Could you check a few things on this model? Use its own coordinates, in mm. Face numbers are marked on the shaded views. A direction names the side the tool comes from. Coordinates: 2 decimals unless noted, no trailing zeros. Loops run counter-clockwise (first coordinate to the right, second up) from the corner with the lowest first, then second, coordinate; pieces in that order, holes last.
1) Will these pins go through, and if not, where does the flat tip stop? P1, Ø6, axis at x = 47, z = 15, coming from the -Y side; P2, Ø14.5, axis at y = -20.5, z = 7, coming from the -X side; P3, Ø6, axis at x = 19.5, y = -26.5, coming from the +Z side; P4, Ø4, axis at x = 47.5, z = 4.5, coming from the -Y side.
2) Thinking about a two-plate mould opening in X: for the marked faces 4, 5 and 6, which applies, released by +X, released by -X, zero draft, split by the parting line, or undercut?
3) Imagine slicing it at B-B on x = 20.5. Please give me the cut outline in (y, z), plus the area to 3 significant figures.
4) For the marked faces 1, 2 and 3, which set-ups out of +Z, -Z, +X, -X, +Y, -Y let a thin tool reach every point of the face, with its end or its side?
5) If I drill on line 1 along Y through (x, z) = (10.5, 13.5); line 2 along X through (y, z) = (-9, 4.5); line 3 along X through (y, z) = (-27.5, -0.5), over which ranges is the centre line in solid material (lowest first)?
6) Imagine slicing it at D-D on y = -20. Please give me the cut outline in (x, z).
7) Imagine slicing it at C-C on z = -0.5. Please give me the cut outline in (x, y).
```python
from build123d import *

# Parameters (mm, degrees)
F0_W     = 52
F0_H     = 32
F1_DEPTH = 40
F2_R     = 15.99999
F3_R     = 8
F4_DEPTH = 40.001
F5_W     = 26.99999
F5_H     = 18
F5_W_2   = 25.00001
F6_DEPTH = 32.001
F7_R     = 9
F8_DEPTH = 32


# Not quite as in the source:
# - a fillet or chamfer is up to 0.001 mm smaller than in the source, because OpenCascade refuses the exact size


with BuildPart() as f1:
    # F0 (on Front) → F1 (new body)
    with BuildSketch(Plane.XZ):
        with Locations((6.3565019518, 4.5450745088)):
            Rectangle(F0_W, F0_H)
    extrude(amount=F1_DEPTH)

    # F2 (radius 16 in the source; OpenCascade refuses exactly that, so slightly less here)
    f2_edges = [f1.edges().sort_by_distance(p)[0] for p in [
        (-19.643498, -20, 20.545075),
        (-19.643498, -20, -11.454925),
    ]]
    fillet(f2_edges, radius=F2_R)

    # F3 (on face) → F4 (cut, through all)
    with BuildSketch(Plane.XZ.offset(40)):
        with Locations((-3.6434980482, 4.5450745088)):
            Circle(F3_R)
    extrude(amount=-F4_DEPTH, mode=Mode.SUBTRACT)

    # F5 (on face) → F6 (cut, through all)
    with BuildSketch(Plane.XY.offset(20.5450745088)):
        with Locations((-17.1435030482, -20)):
            Rectangle(F5_W, F5_H)
        with Locations((8.8564969518, -20)):
            Rectangle(F5_W_2, F5_H)
    extrude(amount=-F6_DEPTH, mode=Mode.SUBTRACT)

    # F7 (on face) → F8 (join)
    with BuildSketch(Plane.YZ.offset(32.3565019518)):
        with Locations((-20, 4.5450745088)):
            Circle(F7_R)
    extrude(amount=F8_DEPTH)


solid = f1.part
```
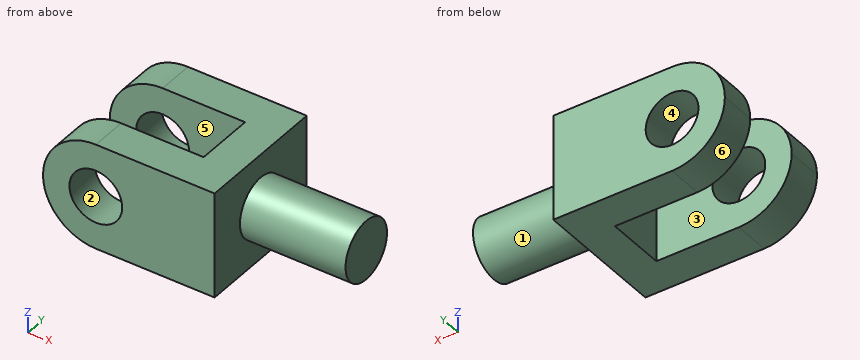
Filled in:
1. P1: stops at y = -25.04
1. P2: stops at x = 21.36
1. P3: stops at z = 20.55
1. P4: stops at y = -29
2. face 4: undercut
2. face 5: zero draft
2. face 6: released by -X
3. outline: (-40, -11.45) - (-29, -11.45) - (-29, 20.55) - (-40, 20.55) - close; (-11, -11.45) - (0, -11.45) - (0, 20.55) - (-11, 20.55) - close
3. area: 704 mm2
4. face 1: +X
4. face 2: +Y, -Y
4. face 3: +Z, -Z, -X
5. line 1: y = -40 to -29, -11 to 0
5. line 2: x = -19.64 to -11.64, 4.36 to 32.36
5. line 3: x = 21.36 to 32.36
6. outline: (21.36, -11.45) - (32.36, -11.45) - (32.36, -4.45) - (64.36, -4.45) - (64.36, 13.55) - (32.36, 13.55) - (32.36, 20.55) - (21.36, 20.55) - close
7. outline: (-18.83, -40) - (-9.85, -40) - (-9.85, -29) - (-18.83, -29) - close; (-18.83, -11) - (-9.85, -11) - (-9.85, 0) - (-18.83, 0) - close; (2.57, -40) - (32.36, -40) - (32.36, -27.45) - (64.36, -27.45) - (64.36, -12.55) - (32.36, -12.55) - (32.36, 0) - (2.57, 0) - (2.57, -11) - (21.36, -11) - (21.36, -29) - (2.57, -29) - close
